Check sheet for the modelled part. Datum: model origin and axes. Units: mm. A direction names the side the tool comes from. Round coordinates to 2 decimals unless told otherwise and drop trailing zeros. Write each loop counter-clockwise with the first axis right and the second up, starting at its lowest first coordinate (ties: lowest second). Pieces come first, ordered by that corner, then holes. Notation, with made-up numbers: (8, 3) -> (44, 3) arc R9 ccw to (44, 9) -> close; hole circle Ø6 at (59, 23). An arc over 180 degrees is marked (long way). Use one line per item in the form item = value. Start each with the question number.
```python
from build123d import *

# Parameters (mm, degrees)
CUT_EXTRUDE_1_DEPTH = 0.5
FILLET_1_R          = 0.5


with BuildPart() as part:
    # 草图1 → 旋转1 (revolve)
    with BuildSketch(Plane.XY):
        Polygon((0, 0), (0, 2.05), (1.38, 2.05), (1.38, 1), (8.38, 1), (9.38, 0), align=None)
    revolve(axis=Axis((-6.976540153, 0, 0), (1, 0, 0)))

    # 草图2 → 切除-拉伸1 (cut)
    with BuildSketch(Plane.ZY):
        Polygon((-0.3, 0.3), (-1, 0.3), (-1, -0.3), (-0.3, -0.3), (-0.3, -1), (0.3, -1), (0.3, -0.3), (1, -0.3), (1, 0.3), (0.3, 0.3), (0.3, 1), (-0.3, 1), align=None)
    extrude(amount=-CUT_EXTRUDE_1_DEPTH, mode=Mode.SUBTRACT)

    # 圆角1
    fillet_1_edges = [part.edges().sort_by_distance(p)[0] for p in [
        (0, -2.05, 0),
    ]]
    fillet(fillet_1_edges, radius=FILLET_1_R)


solid = part.part
```
1. Depth check by flat-ended pin: pin 1 (2 mm diameter, centred on x = 5.5, y = 1, fed in from +Z); pin 2 (0.6 mm diameter, centred on x = 0, z = -1, fed in from +Y); pin 3 (0.6 mm diameter, centred on x = 0.5, z = 0.5, fed in from -Y). Enter the tip coordinate at first touch or a pass-through.
2. Mould release check, pull along Z, two halves, no side actions. Record for faces 3 (the face through (9.109, -0.059, -0.264)), 4 (the face through (0.5, 0, 0)): +Z half, -Z half, draft (parallel to the pull), parting line (faces both ways), or undercut.
3. Tool access check on faces 1 (the face through (5, 0, -1)), 2 (the face through (0.946, -0.267, 2.033)). Record the directions out of +Z, -Z, +X, -X, +Y, -Y that give a thin tool (end or side, any length) a straight path to the whole face; none if there is none.
4. Sectioned sample at A-A (x = 7). Enter the section's corners in (y, z).
5. Scan lines: probe 1 along X at (y, z) = (-0.9, 0.5); probe 2 along Z at (x, y) = (4, 0.55); probe 3 along Y at (x, z) = (8, 0.15). Record each from-to range of solid material in increasing order.
Returned:
q1.pin_1 = 1
q1.pin_2 = 1.8
q1.pin_3 = -2.04
q2.face_3 = parting line
q2.face_4 = undercut
q3.face_1 = +X
q3.face_2 = +X, -X
q4.outline = circle Ø2 at (0, 0)
q5.probe_1 = 0 to 1.38
q5.probe_2 = -0.84 to 0.84
q5.probe_3 = -0.99 to 0.99
